from build123d import *

# Parameters (mm, degrees)
SKETCH1_R           = 4
SKETCH1_R_2         = 1.75
BOSS_EXTRUDE1_DEPTH = 7
SKETCH2_R           = 2.875
CUT_EXTRUDE1_DEPTH  = 5
CUT_EXTRUDE3_REACH  = 35.245
SKETCH4_W           = 13.65685425
SKETCH4_H           = 6.828427125
SKETCH5_R           = 2.875
BOSS_EXTRUDE2_DEPTH = 0.8
FILLET1_R           = 3


with BuildPart() as part:
    # Sketch1 → Boss-Extrude1 (new body)
    # profile 1 of 3: a face of its own
    with BuildSketch(Plane(origin=(0, 0, 0), x_dir=(1, 0, 0), z_dir=(0, 1, 0))):
        with Locations((-17, 8.809397513)):
            Circle(SKETCH1_R)
        with Locations(Location((-17, 8.809397513, 0), (0, 0, 270))):
            Circle(SKETCH1_R_2, mode=Mode.SUBTRACT)
    # profile 2 of 3: a face of its own
    with BuildSketch(Plane(origin=(0, 0, 0), x_dir=(1, 0, 0), z_dir=(0, 1, 0))):
        with Locations((17, 8.809397513)):
            Circle(SKETCH1_R)
        with Locations(Location((17, 8.809397513, 0), (0, 0, 270))):
            Circle(SKETCH1_R_2, mode=Mode.SUBTRACT)
    # profile 3 of 3: a face of its own
    with BuildSketch(Plane(origin=(0, 0, 0), x_dir=(1, 0, 0), z_dir=(0, 1, 0))):
        Polygon((-22.980970389, 0), (0, -22.980970389), (22.980970389, 0), (0, 22.980970389), align=None)
        Polygon((-20.152543264, 0), (0, -20.152543264), (20.152543264, 0), (0, 20.152543264), align=None, mode=Mode.SUBTRACT)
    extrude(amount=BOSS_EXTRUDE1_DEPTH)

    # Sketch2 → Cut-Extrude1 (cut)
    with BuildSketch(Plane(origin=(0, 7, 0), x_dir=(1, 0, 0), z_dir=(0, 1, 0))):
        with Locations(Location((-17, 8.809397513, 0), (0, 0, 270))):
            Circle(SKETCH2_R)
        with Locations(Location((17, 8.809397513, 0), (0, 0, 270))):
            Circle(SKETCH2_R)
    extrude(amount=-CUT_EXTRUDE1_DEPTH, mode=Mode.SUBTRACT)

    # Sketch4 → Cut-Extrude3 (cut, up to next)
    with BuildSketch(Plane(origin=(0, 7, 0), x_dir=(1, 0, 0), z_dir=(0, 1, 0)), mode=Mode.PRIVATE) as cut_extrude3_sk1:
        with Locations((0, 19.566756827)):
            Rectangle(SKETCH4_W, SKETCH4_H)
    cut_extrude3_tool1 = extrude(cut_extrude3_sk1.sketch, amount=-CUT_EXTRUDE3_REACH, mode=Mode.PRIVATE) & part.part
    add(cut_extrude3_tool1.solids().sort_by_distance((0, 7, -19.566757))[0], mode=Mode.SUBTRACT)

    # Sketch5 → Boss-Extrude2 (add)
    # profile 1 of 2: a face of its own
    with BuildSketch(Plane(origin=(0, 7, 0), x_dir=(1, 0, 0), z_dir=(0, 1, 0))):
        with BuildLine():
            Line((13.136296695, 9.844673694), (6.828427125, 16.152543264))
            Line((6.828427125, 16.152543264), (4, 16.152543264))
            Line((4, 16.152543264), (20.152543264, 0))
            Line((20.152543264, 0), (0, -20.152543264))
            Line((0, -20.152543264), (-20.152543264, 0))
            Line((-20.152543264, 0), (-4, 16.152543264))
            Line((-4, 16.152543264), (-6.828427125, 16.152543264))
            Line((-6.828427125, 16.152543264), (-13.136296695, 9.844673694))
            ThreePointArc((-13.136296695, 9.844673694), (-19.828427125, 11.637824638), (-18.03527618, 4.945694208))
            Line((-18.03527618, 4.945694208), (-22.980970389, 0))
            Line((-22.980970389, 0), (0, -22.980970389))
            Line((0, -22.980970389), (22.980970389, 0))
            Line((22.980970389, 0), (18.03527618, 4.945694208))
            ThreePointArc((18.03527618, 4.945694208), (19.828427125, 11.637824638), (13.136296695, 9.844673694))
        make_face()
        with Locations(Location((17, 8.809397513, 0), (0, 0, 270))):
            Circle(SKETCH5_R, mode=Mode.SUBTRACT)
        with Locations(Location((-17, 8.809397513, 0), (0, 0, 270))):
            Circle(SKETCH5_R, mode=Mode.SUBTRACT)
    # profile 2 of 2: a face of its own
    with BuildSketch(Plane(origin=(0, 7, 0), x_dir=(1, 0, 0), z_dir=(0, 1, 0))):
        Polygon((-4, 16.152543264), (4, 16.152543264), (20.152543264, 0), (0, -20.152543264), (-20.152543264, 0), align=None)
    extrude(amount=BOSS_EXTRUDE2_DEPTH)

    # Fillet1
    fillet1_edges = [part.edges().sort_by_distance(p)[0] for p in [
        (22.980970389, 3.9, 0),
        (0, 3.9, 22.980970389),
        (-22.980970389, 3.9, 0),
        (6.828427125, 3.9, -16.152543264),
        (-6.828427125, 3.9, -16.152543264),
    ]]
    fillet(fillet1_edges, radius=FILLET1_R)


solid = part.part
Here's how the part is built. I have some questions about the finished solid (model axes, mm). A direction names the side the tool comes from. Coordinates: 2 decimals unless noted, no trailing zeros. Loops run counter-clockwise (first coordinate to the right, second up) from the corner with the lowest first, then second, coordinate; pieces in that order, holes last. Notation, with made-up numbers: (9.5, 1) -> (34.5, 1) arc R18 cw to (34.5, 32) -> close; hole circle Ø9 at (5, -38). An arc over 180 degrees is marked (long way). Use one line per item in the form item = value. Start each with the question number.
(1) Will these pins go through, and if not, where does the flat tip stop? pin 1 (3 mm diameter, centred on x = 4, z = -11, fed in from -Y); pin 2 (4.5 mm diameter, centred on x = -17, z = -8.81, fed in from +Y); pin 3 (4 mm diameter, centred on x = -8, y = 2, fed in from -Z); pin 4 (3 mm diameter, centred on x = 17, z = -8.81, fed in from +Y).
(2) If we section it at B-B (x = -17): Please give me the cut outline in (y, z).
(3) If we section it at A-A (y = 5.5): Please give me the cut outline in (x, z) (3 decimals), then the cut area to 3 significant figures.
(4) If we section it at C-C (z = 16.5): Please give me the cut outline in (x, y), then the cut area to 3 significant figures.
(5) If we section it at D-D (x = 7): Please give me the cut outline in (y, z).
(6) We'd pull the mould along X, two halves only. Please class faces 6 (the face through (10, 0, 11)), 7 (the face through (-10.38, 3.85, -12.6)), 8 (the face through (0.03, 3.85, 21.74)), 9 (the face through (6.749, 3.845, -15.918)): pulls with the +X half, pulls with the -X half, needs draft (parallel to the pull), parting line crosses it, or undercut.
(7) On a 3-axis mill with a long thin cutter (end or side, diameter ignored), from which of +Z, -Z, +X, -X, +Y, -Y can I reach the whole of each face in a straight line? I mean faces 1 (the face through (0, 7, 2)), 2 (the face through (10.46, 3.85, -12.52)), 3 (the face through (14.193, 4.859, -9.433)), 4 (the face through (-11.62, 3.85, 11.36)), 5 (the face through (-15.265, 0.986, -9.037)). Say none if no direction works.
(8) Please list where these lines run through material, in increasing order: line 1 along Z through (x, y) = (17, 1.2); line 2 along X through (y, z) = (5.75, -12); line 3 along Y through (x, z) = (-13.5, -2).
Verdict:
q1.pin_1 = 7
q1.pin_2 = 2
q1.pin_3 = -16.12
q1.pin_4 = through
q2.outline = (0, -12.81) -> (7.8, -12.81) -> (7.8, -11.68) -> (2, -11.68) -> (2, -10.56) -> (0, -10.56) -> close; (0, -7.06) -> (2, -7.06) -> (2, -5.93) -> (7.8, -5.93) -> (7.8, 5.98) -> (0, 5.98) -> (0, 3.15) -> (7, 3.15) -> (7, -3.15) -> (0, -3.15) -> close
q3.outline = (-20.86, -2.121) -> (-18.035, -4.946) arc R4 ccw (long way) to (-13.136, -9.845) -> (-7.707, -15.274) arc R3 ccw to (-5.586, -16.153) -> (-4, -16.153) -> (-20.153, 0) -> (0, 20.153) -> (20.153, 0) -> (4, -16.153) -> (5.586, -16.153) arc R3 ccw to (7.707, -15.274) -> (13.136, -9.845) arc R4 ccw (long way) to (18.035, -4.946) -> (20.86, -2.121) arc R3 ccw to (20.86, 2.121) -> (2.121, 20.86) arc R3 ccw to (-2.121, 20.86) -> (-20.86, 2.121) arc R3 ccw to start; hole circle Ø5.75 at (-17, -8.809); hole circle Ø5.75 at (17, -8.809)
q3.area = 236 mm²
q4.outline = (-6.48, 0) -> (-3.65, 0) -> (-3.65, 7) -> (3.65, 7) -> (3.65, 0) -> (6.48, 0) -> (6.48, 7.8) -> (-6.48, 7.8) -> close
q4.area = 50.0 mm²
q5.outline = (0, -15.8) -> (7.8, -15.8) -> (7.8, 15.98) -> (0, 15.98) -> (0, 13.15) -> (7, 13.15) -> (7, -13.15) -> (0, -13.15) -> close
q6.face_6 = needs draft
q6.face_7 = undercut
q6.face_8 = parting line crosses it
q6.face_9 = pulls with the +X half
q7.face_1 = -Y
q7.face_2 = -Z, +Y, -Y
q7.face_3 = +Y
q7.face_4 = +Z, -X, +Y, -Y
q7.face_5 = +Y, -Y
q8.line_1 = -12.81 to -10.56, -7.06 to -3.15, 3.15 to 5.98
q8.line_2 = -19.41 to -14.59, -10.98 to -8.15, 8.15 to 10.98, 14.59 to 19.41
q8.line_3 = 7 to 7.8
